Source: CAD feature listing. Evaluate the final solid. Frame: model axes, mm. Round coordinates to 2 decimals unless told otherwise and drop trailing zeros. Order: outer loops, then holes, each group sorted by start corner. A loop starts at its lowest first (then second) coordinate and runs counter-clockwise, first axis right, second up. Notation, with made-up numbers: (0, -16) - (42, -16) arc R23 cw to (42, 19) - close; hole circle Ø6 at (83.25, 7). An arc over 180 degrees is marked (long way). Return JSON: item names as keys, results as strings. Group by question number.
1) Contact query for a flat-ended pin moving along its axis: P1, Ø8, axis at y = -29, z = -14, coming from the +X side. Output: stop coordinate, or through.
2) Section B-B, the plane z = -13.25. Return loops of the section in (x, y).
3) Ray query, line 1 (X direction, y = -4.5, z = -5); line 2 (X direction, y = -25.5, z = -16.25); line 3 (Z direction, x = 1.75, y = -26.5). Return the intervals inside material, ascending. Write a range as from..to.
4) Section A-A, the plane y = -6.5. Return loops of the section in (x, z), plus the area to 3 significant figures.
5) Section C-C, the plane x = 1. Return loops of the section in (y, z).
```python
from build123d import *

# Parameters (mm, degrees)
F1_DEPTH = 40
F2_W     = 5
F2_H     = 18.6602540378
F3_DEPTH = 40.001
F4_R     = 2


with BuildPart() as f1:
    # F0 (on Front) → F1 (new body)
    with BuildSketch(Plane.XZ):
        Polygon((10.7179676972, 0), (0, 0), (0, -40), align=None)
    extrude(amount=F1_DEPTH)

    # F2 (on face) → F3 (cut, through all)
    with BuildSketch(Plane.XZ.offset(40)):
        with Locations((2.5, -30.6698729811)):
            Rectangle(F2_W, F2_H)
    extrude(amount=-F3_DEPTH, mode=Mode.SUBTRACT)

    # F4
    f4_edges = [f1.edges().sort_by_distance(p)[0] for p in [
        (0, -20, 0),
        (0, -20, -21.339746),
    ]]
    fillet(f4_edges, radius=F4_R)


solid = f1.part
```
Geometry check:
{
 "1": {"P1": "x = 8.04"},
 "2": {"outline": "(0, -40) - (7.17, -40) - (7.17, 0) - (0, 0) - close"},
 "3": {"line 1": "0..9.38", "line 2": "0..6.36", "line 3": "-21.32..-0.02"},
 "4": {"outline": "(0, -19.34) arc R2 ccw to (2, -21.34) - (5, -21.34) - (10.72, 0) - (2, 0) arc R2 ccw to (0, -2) - close", "area": "166 mm2"},
 "5": {"outline": "(-40, -21.07) - (0, -21.07) - (0, -0.27) - (-40, -0.27) - close"}
}
